Work out the finished part from the listing and answer in its coordinate system (mm). Face numbers are marked on the shaded views. A direction names the side the tool comes from. Coordinates: 2 decimals unless noted, no trailing zeros. Order: outer loops, then holes, each group sorted by start corner. A loop starts at its lowest first (then second) coordinate and runs counter-clockwise, first axis right, second up. Notation, with made-up numbers: M -23,1.5 L 23,1.5 A29 cw 23,33.5 Z; hole C 53,17.25 d4. An arc over 180 degrees is marked long. Write item = value, one per line. Start each with the question number.
Q1. Find section A-A on x = 1.5. Give the vertices of the cut face in (y, z).
Q2. Straight lines are drawn through the part: line 1 along Z through (x, y) = (-32.5, 87); line 2 along X through (y, z) = (45, 1.5); line 3 along Z through (x, y) = (39, 34). For each, find the intervals that lie inside material, in ascending order.
Q3. A tool of negligible diameter and unlimited length cuts with its end or side. For the marked faces 5 and 6, from which of +Z, -Z, +X, -X, +Y, -Y can it reach the whole face along a straight path? Write none if from no direction.
Q4. Find section B-B on y = 58. Give the vertices of the cut face in (x, z).
Q5. Find section C-C on x = -39.5. Give the vertices of the cut face in (y, z), and give its area (3 significant figures).
Q6. Determine the mould class of the marked faces 1, 2, 3 and 4 for opening direction X: released by +X, released by -X, zero draft, split by the parting line, or undercut.
Q7. Find section D-D on x = 16. Give the vertices of the cut face in (y, z), and give its area (3 significant figures).
Q8. Each of these flat-tipped pins is pushed along its axis until it touches: P1, Ø7.5, axis at x = 10.5, z = -10.5, coming from the -Y side; P2, Ø16, axis at y = 80, z = -9, coming from the +X side; P3, Ø1, axis at x = 4, y = 21, coming from the -Z side. Where does it stop, or does it pass through?
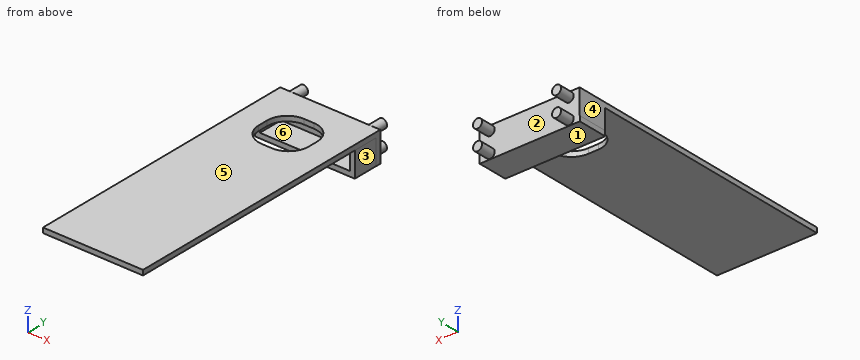
Autodesk Inventor part; units mm, degrees
ref_plane "YZ Plane" through (0, 0, 0) normal (1, 0, 0) x (0, 1, 0)
ref_plane "XZ Plane" through (0, 0, 0) normal (0, 1, 0) x (-1, 0, 0)
ref_plane "XY Plane" through (0, 0, 0) normal (0, 0, 1) x (1, 0, 0)
sketch "Sketch1" plane through (0, 0, 0) normal (0, 0, 1) x (1, 0, 0)
  line L0 (-50, -100) -> (50, -100)
  line L1 (50, -100) -> (50, 100)
  line L2 (50, 100) -> (-50, 100)
  line L3 (-50, 100) -> (-50, -100)
  line L4 (-50, -100) -> (50, 100) construction
  line L5 (50, -100) -> (-50, 100) construction
  point P0 (0, 0)
  dimension "d0" = 100
  dimension "d1" = 200
extrude "Extrusion1" add sketch "Sketch1" along normal blind 5
sketch "Sketch6" plane through (0, 0, 5) normal (0, 0, 1) x (1, 0, 0)
  line L0 (4.9986, 75) -> (-5.0014, 75)
  line L1 (-25.0014, 55) -> (-25.0014, 45)
  line L2 (-5.0014, 25) -> (4.9986, 25)
  line L3 (24.9986, 45) -> (24.9986, 55)
  line L4 (24.9986, 75) -> (-25.0014, 25) construction
  line L5 (-25.0014, 75) -> (24.9986, 25) construction
  arc A0 (4.9986, 25) -> (24.9986, 45) centre (4.9986, 45) ccw
  arc A1 (24.9986, 55) -> (4.9986, 75) centre (4.9986, 55) ccw
  arc A2 (-5.0014, 75) -> (-25.0014, 55) centre (-5.0014, 55) ccw
  arc A3 (-25.0014, 45) -> (-5.0014, 25) centre (-5.0014, 45) ccw
  point P0 (0, 0)
  point P1 (-0.0014, 50)
  dimension "d21" = 50
  dimension "d22" = 50
  dimension "d23" = 20
extrude "Extrusion6" cut sketch "Sketch6" against normal blind 5
sketch "Sketch15" plane through (-50, 100, 5) normal (0, 1, 0) x (1, 0, 0)
  line L0 (100, 0) -> (0, 0)
  line L1 (0, 0) -> (100, 0)
  line L2 (100, 0) -> (100, 30)
  line L3 (100, 30) -> (0, 30)
  line L4 (0, 30) -> (0, 0)
  point P0 (50, 5)
  dimension "d46" = 100
  dimension "d47" = 30
sketch "Sketch16" plane through (-50, 100, 5) normal (0, 1, 0) x (1, 0, 0)
  circle A0 centre (10.5, 5) radius 4.5
  circle A1 centre (89.5, 5) radius 4.5
  circle A2 centre (10.5, 25) radius 4.5
  circle A3 centre (89.5, 25) radius 4.5
  point P0 (50, 5)
  dimension "d48" = 9
  dimension "d49" = 9
  dimension "d50" = 9
  dimension "d51" = 9
extrude "Extrusion11" add sketch "Sketch15" against normal blind 5
extrude "Extrusion12" add sketch "Sketch16" along normal blind 15
sketch "Sketch17" plane through (50, 100, -25) normal (0, 0, -1) x (-1, 0, 0)
  line L0 (100.0829, 0) -> (0.0829, 0)
  line L1 (0.0829, 0) -> (0.0829, -30)
  line L2 (0.0829, -30) -> (100.0829, -30)
  line L3 (100.0829, -30) -> (100.0829, 0)
  point P0 (50, -100)
  dimension "d56" = 100
  dimension "d57" = 30
extrude "Extrusion13" add sketch "Sketch17" against normal blind 5
sketch "Sketch18" plane through (49.9171, 70, -25) normal (1, 0, 0) x (0, 0, -1)
  line L0 (0, 0) -> (-5, 0)
  line L1 (-30, 30) -> (-30, -170)
  line L2 (0, 0) -> (-30, 0)
  line L3 (-30, 0) -> (-30, 30)
  line L4 (-30, 30) -> (0, 30)
  line L5 (0, 30) -> (0, 0)
  point P0 (-25, -70)
extrude "Extrusion14" add sketch "Sketch18" against normal blind 5
sketch "Sketch20" plane through (-50, -100, 5) normal (-1, 0, 0) x (0, 0, 1)
  line L0 (-30, 200) -> (0, 200)
  line L1 (-30, 170) -> (-30, 200)
  line L2 (0, 200) -> (-30, 200)
  line L3 (-30, 200) -> (-30, 170)
  line L4 (-30, 170) -> (0, 170)
  line L5 (0, 170) -> (0, 200)
  point P0 (-5, 100)
extrude "Extrusion16" add sketch "Sketch20" against normal blind 5
sketch "Sketch21" plane through (0, 0, 5) normal (0, 0, 1) x (1, 0, 0)
  line L0 (50, -100) -> (50, 100)
  line L1 (50, -100) -> (-50, -100)
  line L2 (-50, -100) -> (-50, -180)
  line L3 (-50, -180) -> (50, -180)
  line L4 (50, -180) -> (50, -100)
  point P0 (0, 0)
  dimension "d66" = 100
  dimension "d67" = 80
extrude "Extrusion17" add sketch "Sketch21" against normal blind 5
properties part number "fixation_v03"
Findings below:
q1.outline = M -180,0 L 25,0 L 25,5 L -180,5 Z; M 70,-25 L 100,-25 L 100,5 L 75,5 L 75,0 L 95,0 L 95,-20 L 70,-20 Z
q2.line_1 = -25 to -20, 0 to 5
q2.line_2 = -50 to -25, 25 to 50
q2.line_3 = 0 to 5
q3.face_5 = +Z, +X, -X, +Y, -Y
q3.face_6 = -Y
q4.outline = M -50,0 L -24.78,0 L -24.78,5 L -50,5 Z; M 24.77,0 L 50,0 L 50,5 L 24.77,5 Z
q5.outline = M -180,0 L 95,0 L 95,-20 L 70,-20 L 70,-25 L 100,-25 L 100,-24.5 L 115,-24.5 L 115,-15.5 L 100,-15.5 L 100,-4.5 L 115,-4.5 L 115,4.5 L 100,4.5 L 100,5 L -180,5 Z
q5.area = 1,920 mm^2
q6.face_1 = zero draft
q6.face_2 = undercut
q6.face_3 = released by +X
q6.face_4 = released by -X
q7.outline = M -180,0 L 28.3,0 L 28.3,5 L -180,5 Z; M 70,-25 L 100,-25 L 100,5 L 71.7,5 L 71.7,0 L 95,0 L 95,-20 L 70,-20 Z
q7.area = 1,430 mm^2
q8.P1 = 95
q8.P2 = 49.92
q8.P3 = 0
